Read the model definition and answer for the solid it produces. Units are mm, in the model's axes. A direction names the side the tool comes from. Give positions to 0.01 mm unless a question says otherwise; leave off trailing zeros. Loops run counter-clockwise (first coordinate to the right, second up) from the corner with the lowest first, then second, coordinate; pieces in that order, holes last. Notation, with made-up numbers: (46, -19.5) - (63, -19.5) arc R26 cw to (63, 2.5) - close; hole circle Ø7 at (11, -7.75). An arc over 180 degrees is marked (long way). Write each question's results on one line, items separated by ' | '. Start each with the question number.
Q1. The part is cut by section A-A, the plane x = 10. Write down the section's boundary in (y, z).
Q2. Determine the mould class of faces 4 (the flat face through (0, -17, 12)), 5 (the flat face through (-5, -10, 25)), 6 (the cylindrical face through (8.91, -7.6, 25.09)), 7 (the flat face through (5, -8, 0)) for opening direction Z: +Z half, -Z half, draft (parallel to the pull), parting line (faces both ways), or undercut.
Q3. The part is cut by section B-B, the plane z = 10. Write down the section's boundary in (x, y).
Q4. Given pin 1 (3 mm diameter, centred on x = -7, y = -7, fed in from +Z); pin 2 (9 mm diameter, centred on x = 10, z = 10, fed in from -Y); pin 3 (1.5 mm diameter, centred on y = -17.5, z = 9.5, fed in from +X); pin 4 (6 mm diameter, centred on x = 9.5, z = 19, fed in from -Y), each flat-ended and moving along its own axis, determine where each tip first touches the part or whether it passes through.
Q5. For faces 1 (the flat face through (0, -7, 33)), 2 (the flat face through (5, 0, 20)), 3 (the flat face through (10, -15, 20)), determine the directions among +Z, -Z, +X, -X, +Y, -Y from which every point of the face is accessible in a straight line to the end or side of a thin tool.
Q6. The part is cut by section D-D, the plane z = 22.5. Write down the section's boundary in (x, y), plus the area to 3 significant figures.
Q7. Find the intervals of material crossed by line 1 (Z direction, x = 10, y = -4); line 2 (Y direction, x = 2, z = 17.5); line 3 (X direction, y = -10.5, z = 7), in increasing order. Write a range as from..to.
Q8. The part is cut by section C-C, the plane y = -2.25. Write down the section's boundary in (x, z), plus the area to 3 significant figures.
```python
from build123d import *

# Parameters (mm, degrees)
F1_DEPTH = 15
F0_W     = 10
F0_H     = 25
F2_DEPTH = 20
F3_R     = 5
F3_R_2   = 5.029307
F4_DEPTH = 15


with BuildPart() as f1:
    # F0 (on Front) → F1 (new body)
    with BuildSketch(Plane.XZ):
        Polygon((0, 25), (0, 0), (20, 0), (20, 40), (0, 40), align=None)
    extrude(amount=F1_DEPTH)

    # F0 (on Front) → F2 (join)
    with BuildSketch(Plane.XZ):
        with Locations((-5, 12.5)):
            Rectangle(F0_W, F0_H)
    extrude(amount=F2_DEPTH)

    # F3 (on face) → F4 (cut)
    with BuildSketch(Plane.XZ.offset(15)):
        with Locations((10, 10)):
            Circle(F3_R)
        with Locations((10, 30)):
            Circle(F3_R_2)
    extrude(amount=-F4_DEPTH, mode=Mode.SUBTRACT)


solid = f1.part
```
Check sheet entries:
1) outline: (-15, 0) - (0, 0) - (0, 5) - (-15, 5) - close; (-15, 15) - (0, 15) - (0, 24.97) - (-15, 24.97) - close; (-15, 35.03) - (0, 35.03) - (0, 40) - (-15, 40) - close
2) face 4: draft | face 5: +Z half | face 6: undercut | face 7: -Z half
3) outline: (-10, -20) - (0, -20) - (0, -15) - (5, -15) - (5, 0) - (-10, 0) - close; (15, -15) - (20, -15) - (20, 0) - (15, 0) - close
4) pin 1: stops at z = 25 | pin 2: passes through | pin 3: stops at x = 0 | pin 4: stops at y = -15
5) face 1: +Z, -X, +Y, -Y | face 2: +Z, -Z, +X, -X, +Y | face 3: +Z, -Z, +X, -Y
6) outline: (-10, -20) - (0, -20) - (0, -15) - (20, -15) - (20, 0) - (-10, 0) - close | area: 500 mm^2
7) line 1: z = 0..5, 15..24.97, 35.03..40 | line 2: y = -15..0 | line 3: x = -10..6, 14..20
8) outline: (-10, 0) - (20, 0) - (20, 40) - (0, 40) - (0, 25) - (-10, 25) - close; hole circle Ø10.06 at (10, 30); hole circle Ø10 at (10, 10) | area: 892 mm^2
